from build123d import *

# Parameters (mm, degrees)
F0_W     = 50.8
F0_H     = 31.75
F1_DEPTH = 12.7
F2_W     = 50.8
F2_H     = 19.05
F3_DEPTH = 12.7
F5_DEPTH = 25.4
F6_W     = 9.14671
F6_H     = 19.05
F7_DEPTH = 19.05
F9_DEPTH = 25.4


with BuildPart() as f1:
    # F0 (on Top) → F1 (new body)
    with BuildSketch(Plane.XY):
        with Locations((-7.10658, 15.875)):
            Rectangle(F0_W, F0_H)
    extrude(amount=F1_DEPTH)

    # F2 (on face) → F3 (join)
    with BuildSketch(Plane.XZ):
        with Locations((-7.10658, 22.225)):
            Rectangle(F2_W, F2_H)
    extrude(amount=-F3_DEPTH)

    # F4 (on face) → F5 (cut)
    with BuildSketch(Plane.XZ):
        Polygon((18.29342, 31.75), (0, 31.75), (18.29342, 12.7), align=None)
    extrude(amount=-F5_DEPTH, mode=Mode.SUBTRACT)

    # F6 (on face) → F7 (join)
    with BuildSketch(Plane(origin=(0, 12.7, 0), x_dir=(-1, 0, 0), z_dir=(0, 1, 0))):
        with Locations((11.679935, 22.225)):
            Rectangle(F6_W, F6_H)
    extrude(amount=F7_DEPTH)

    # F8 (on face) → F9 (cut)
    with BuildSketch(Plane.YZ.offset(-7.10658)):
        Polygon((31.75, 31.75), (12.7, 31.75), (31.75, 12.7), align=None)
    extrude(amount=-F9_DEPTH, mode=Mode.SUBTRACT)


solid = f1.part
Build history of the part. All positions in model axes, mm. A direction names the side the tool comes from. Round coordinates to 2 decimals unless told otherwise and drop trailing zeros. Write each loop counter-clockwise with the first axis right and the second up, starting at its lowest first coordinate (ties: lowest second). Pieces come first, ordered by that corner, then holes. Notation, with made-up numbers: (-23.5, -10) - (-15.5, -10) arc R28 ccw to (-15.5, 10) - close; hole circle Ø8 at (27.5, -30.75). An arc over 180 degrees is marked (long way). Use CSV: the item, a comma, the result in double quotes.
(1) Band-saw the part on A-A (y = 13.5). Write the cut outline in (x, z).
Response:
outline,"(-32.51, 0) - (18.29, 0) - (18.29, 12.7) - (-7.11, 12.7) - (-7.11, 30.95) - (-16.25, 30.95) - (-16.25, 12.7) - (-32.51, 12.7) - close"
(2) Band-saw the part on D-D (x = -15). Write the cut outline in (y, z).
Response:
outline,"(0, 0) - (31.75, 0) - (31.75, 12.7) - (12.7, 31.75) - (0, 31.75) - close"
(3) Band-saw the part on B-B (x = -21). Write the cut outline in (y, z), plus the area to 3 significant figures.
Response:
outline,"(0, 0) - (31.75, 0) - (31.75, 12.7) - (12.7, 12.7) - (12.7, 31.75) - (0, 31.75) - close"
area,"645 mm²"
(4) Wall check: line 1 (Y direction, x = -27, z = 17.5); line 2 (X direction, y = 24, z = 14.5). Give the ranges that are in metal, low to high.
Response:
line 1,"0 to 12.7"
line 2,"-16.25 to -7.11"
(5) Band-saw the part on C-C (z = 18.5). Write the cut outline in (x, y).
Response:
outline,"(-32.51, 0) - (12.72, 0) - (12.72, 12.7) - (-7.11, 12.7) - (-7.11, 25.95) - (-16.25, 25.95) - (-16.25, 12.7) - (-32.51, 12.7) - close"
(6) Pin check, flat tips, straight feed: P1, Ø9.5, axis at x = 10.5, z = 20, coming from the +Y side; P2, Ø5, axis at x = 7, y = 26.5, coming from the +Z side; P3, Ø8, axis at y = 26.5, z = 22.5, coming from the -X side. Stop position of each tip, or through.
Response:
P1,"y = 12.7"
P2,"z = 12.7"
P3,"x = -16.25"
(7) 3-axis set-ups, long thin cutter, end or side, ignore diameter. For faces 1 (the flat face through (-16, 6, 31.75)), 2 (the flat face through (-24, 22, 12.7)), 3 (the flat face through (-7.107, 20, 20)): which of +Z, -Z, +X, -X, +Y, -Y reach the whole face in a straight line?
Response:
face 1,"+Z, +X, -X, +Y, -Y"
face 2,"+Z, -X, +Y"
face 3,"+Z, +X, +Y"
